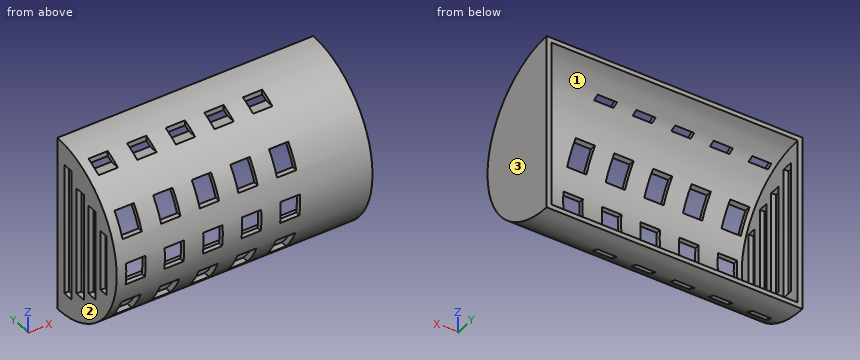
```python
from build123d import *

# Parameters (mm, degrees)
REVOLVE_1_ANGLE     = 180
CUT_EXTRUDE_START   = -100
SKETCH_6_W          = 12.076682438
SKETCH_6_H          = 14.39053984
SKETCH_6_H_2        = 13.782632099
SKETCH_6_H_3        = 13.782632098
SKETCH_6_H_4        = 22.837839873
CUT_EXTRUDE_3_DEPTH = 80
SKETCH_7_W          = 83.279125937
SKETCH_7_H          = 6.800730915
SKETCH_7_W_2        = 68.126620215
SKETCH_7_H_2        = 6.920041983
SKETCH_7_W_3        = 56.91137976
SKETCH_7_H_3        = 6.32348664
SKETCH_7_W_4        = 38.179541977
SKETCH_7_H_4        = 5.488309159
CUT_EXTRUDE_4_DEPTH = 80


with BuildPart() as part:
    # 草图1 → 旋转1 (revolve)
    with BuildSketch(Plane(origin=(0, 0, 0), x_dir=(1, 0, 0), z_dir=(0, 1, 0))):
        Polygon((-78.924564797, 0), (-81.924564797, 0), (-81.924564797, -55.5), (78.075435203, -55.5), (78.075435203, 0), (75.075435203, 0), (75.075435203, -52.5), (-78.924564797, -52.5), align=None)
    revolve(axis=Axis((-95.756286267, 0, 0), (1, 0, 0)), revolution_arc=REVOLVE_1_ANGLE)

    # 草图6 → 切除-拉伸3 (cut)
    with BuildSketch(Plane(origin=(0, 0, 0), x_dir=(1, 0, 0), z_dir=(0, 1, 0)).offset(CUT_EXTRUDE_START)):
        with Locations((-69.886223578, 56.69526992)):
            Rectangle(SKETCH_6_W, SKETCH_6_H)
        with Locations((-69.886223578, 28.826051853)):
            Rectangle(SKETCH_6_W, SKETCH_6_H_2)
        with Locations((-69.886223578, 1.260787656)):
            Rectangle(SKETCH_6_W, SKETCH_6_H_3)
        with Locations((-69.886223578, -26.304476541)):
            Rectangle(SKETCH_6_W, SKETCH_6_H_2)
        with Locations((-69.886223578, -58.397344625)):
            Rectangle(SKETCH_6_W, SKETCH_6_H_4)
        with Locations((-45.732858702, 56.69526992)):
            Rectangle(SKETCH_6_W, SKETCH_6_H)
        with Locations((-21.579493826, 56.69526992)):
            Rectangle(SKETCH_6_W, SKETCH_6_H)
        with Locations((2.57387105, 56.69526992)):
            Rectangle(SKETCH_6_W, SKETCH_6_H)
        with Locations((26.727235926, 56.69526992)):
            Rectangle(SKETCH_6_W, SKETCH_6_H)
        with Locations((-45.732858702, -58.397344625)):
            Rectangle(SKETCH_6_W, SKETCH_6_H_4)
        with Locations((-21.579493826, -58.397344625)):
            Rectangle(SKETCH_6_W, SKETCH_6_H_4)
        with Locations((2.57387105, -58.397344625)):
            Rectangle(SKETCH_6_W, SKETCH_6_H_4)
        with Locations((26.727235926, -58.397344625)):
            Rectangle(SKETCH_6_W, SKETCH_6_H_4)
        with Locations((-45.732858702, 28.826051853)):
            Rectangle(SKETCH_6_W, SKETCH_6_H_2)
        with Locations((-21.579493826, 28.826051853)):
            Rectangle(SKETCH_6_W, SKETCH_6_H_2)
        with Locations((2.57387105, 28.826051853)):
            Rectangle(SKETCH_6_W, SKETCH_6_H_2)
        with Locations((26.727235926, 28.826051853)):
            Rectangle(SKETCH_6_W, SKETCH_6_H_2)
        with Locations((-45.732858702, 1.260787656)):
            Rectangle(SKETCH_6_W, SKETCH_6_H_3)
        with Locations((-21.579493826, 1.260787656)):
            Rectangle(SKETCH_6_W, SKETCH_6_H_3)
        with Locations((2.57387105, 1.260787656)):
            Rectangle(SKETCH_6_W, SKETCH_6_H_3)
        with Locations((26.727235926, 1.260787656)):
            Rectangle(SKETCH_6_W, SKETCH_6_H_3)
        with Locations((26.727235926, -26.304476541)):
            Rectangle(SKETCH_6_W, SKETCH_6_H_2)
        with Locations((2.57387105, -26.304476541)):
            Rectangle(SKETCH_6_W, SKETCH_6_H_2)
        with Locations((-21.579493826, -26.304476541)):
            Rectangle(SKETCH_6_W, SKETCH_6_H_2)
        with Locations((-45.732858702, -26.304476541)):
            Rectangle(SKETCH_6_W, SKETCH_6_H_2)
    extrude(amount=CUT_EXTRUDE_3_DEPTH, mode=Mode.SUBTRACT)

    # 草图7 → 切除-拉伸4 (cut)
    with BuildSketch(Plane.ZY.offset(81.924564797)):
        with Locations((0.238622138, -9.73402863)):
            Rectangle(SKETCH_7_W, SKETCH_7_H)
        with Locations((-0.298277671, -21.366857825)):
            Rectangle(SKETCH_7_W_2, SKETCH_7_H_2)
        with Locations((1.014144084, -32.28382061)):
            Rectangle(SKETCH_7_W_3, SKETCH_7_H_3)
        with Locations((0.95448855, -43.200783394)):
            Rectangle(SKETCH_7_W_4, SKETCH_7_H_4)
    extrude(amount=-CUT_EXTRUDE_4_DEPTH, mode=Mode.SUBTRACT)


solid = part.part
```
Source: CAD feature listing. Evaluate the final solid. Frame: model axes, mm. Face numbers are marked on the shaded views. Give positions to 0.01 mm unless a question says otherwise; leave off trailing zeros. Order: outer loops, then holes, each group sorted by start corner. A loop starts at its lowest first (then second) coordinate and runs counter-clockwise, first axis right, second up.
(1) Section query B-B (y = -11). Return the cut outline in (x, z), plus the area to 3 significant figures.
(2) Material intervals for line 1 along X through (y, z) = (-29, 6); line 2 along Y through (x, z) = (36.5, -8); line 3 along Z through (x, y) = (-21, -14), sorted ascending.
(3) Section query C-C (z = 0). State how many separate pieces and enclosed holes the cut face has, plus the area to 3 significant figures.
(4) Contact query for flat-ended pins moving along their axis: P1, Ø3.5, axis at x = 4.5, y = -49.5, coming from the +Z side; P2, Ø12, axis at x = 0, y = -25, coming from the +Z side; P3, Ø6.5, axis at y = -45.5, z = -32, coming from the +X side; P4, Ø10, axis at x = -10.5, y = -43, coming from the -Z side. Output: stop coordinate, or through.
(5) Section query A-A (x = -25). Return the cut outline in (y, z), plus the area to 3 significant figures.
(6) Pull-direction query (X, two-part tool) for the marked faces 1, 2 and 3; classes: +X half, -X half, draft (parallel to the pull), parting line (faces both ways), or undercut.
Outcome:
1. outline: (-81.92, -54.4) - (78.08, -54.4) - (78.08, 54.4) - (-81.92, 54.4) - (-81.92, 41.88) - (-78.92, 41.88) - (-78.92, 51.33) - (75.08, 51.33) - (75.08, -51.33) - (-78.92, -51.33) - (-78.92, -41.4) - (-81.92, -41.4) - close
1. area: 1,350 mm2
2. line 1: x = -81.92 to -78.92, 75.08 to 78.08
2. line 2: y = -54.92 to -51.89
2. line 3: z = -53.71 to -50.6, 50.6 to 53.71
3. separate pieces: 10
3. enclosed holes: 0
3. area: 537 mm2
4. P1: stops at z = 19.41
4. P2: stops at z = 52.15
4. P3: stops at x = 78.08
4. P4: stops at z = -40.45
5. outline: (-55.21, 5.63) - (-52.2, 5.63) arc R52.5 cw to (-48.78, 19.41) - (-51.99, 19.41) arc R55.5 ccw to start; (-54.9, -8.15) arc R55.5 ccw to (-50.98, -21.93) - (-47.7, -21.93) arc R52.5 cw to (-51.86, -8.15) - close; (-44.48, 33.2) - (-40.67, 33.2) arc R52.5 cw to (-23.44, 46.98) - (-29.55, 46.98) arc R55.5 ccw to start; (-42.48, -35.72) arc R55.5 ccw to (-25.1, -49.5) - (-20, -49.5) - (-20, -51.77) arc R55.5 ccw to (0, -55.5) - (0, -52.5) arc R52.5 cw to (-38.48, -35.72) - close; (-20, 48.54) arc R52.5 cw to (0, 52.5) - (0, 55.5) arc R55.5 ccw to (-20, 51.77) - close
5. area: 342 mm2
6. face 1: undercut
6. face 2: -X half
6. face 3: +X half
